The model under review builds one solid part; all positions refer to its coordinate system, in mm. A direction names the side the tool comes from. Round coordinates to 2 decimals unless told otherwise and drop trailing zeros. Order: outer loops, then holes, each group sorted by start corner. A loop starts at its lowest first (then second) coordinate and runs counter-clockwise, first axis right, second up. Notation, with made-up numbers: M 1,51 L 6,51 A17 cw 6,77 Z; hole C 65.5,63.25 d11. An arc over 180 degrees is marked long. Answer as a JSON object with one key per item and string values. Group by question number.
1. Add section A-A on z = -39.2. State the section outline as (x, y) points.
2. Clearance check with flat-ended pins moving along their axes: P1, Ø6, axis at y = 17.5, z = -7.5, coming from the +X side; P2, Ø1.5, axis at x = 28, z = 1.5, coming from the +Y side; P3, Ø7, axis at x = 1, z = -16, coming from the -Y side; P4, Ø4, axis at y = 1.96, z = -39.2, coming from the -X side. State where each tip first meets the part, or that it passes through.
3. To check wall thickness, follow probe 1 along Y at (x, z) = (-11, -8); probe 2 along Y at (x, z) = (-11, -39); probe 3 along X at (y, z) = (3.5, -15.5). State the ranges of each line that lie inside material, in increasing order. Write a range as [from, to].
4. Mouldability with a two-part tool opening along Y and no side actions: class faces 1 (the face through (1, 25, 3)), 2 (the face through (24, 40.963, 1)), 3 (the face through (-0.37, 32.34, 1.99)), 4 (the face through (7.39, -1.15, 1.48)) as released by +Y, released by -Y, zero draft, split by the parting line, or undercut.
5. Add section B-B on y = 34. State the section outline as (x, z) points, and give its area (3 significant figures).
6. Add section D-D on z = -20. State the section outline as (x, y) points, and give its area (3 significant figures).
7. Machinability: for faces 5 (the face through (-3, 40.963, -7)), 6 (the face through (4.04, 23.95, 1.48)), which of the approach directions +Z, -Z, +X, -X, +Y, -Y give a long, thin tool a straight path to every point of the face, cutting with its end or side? Answer none if there is none.
8. Add section C-C on x = 0. State the section outline as (y, z) points.
```python
from build123d import *

# Parameters (mm, degrees)
SKETCH_1_R          = 1.7
EXTRUDE_1_DEPTH     = 3
SKETCH_2_W          = 3.161086378
SKETCH_2_H          = 42
EXTRUDE_2_DEPTH     = 45
SKETCH_3_R          = 1.7
SKETCH_3_R_2        = 13
CUT_EXTRUDE_1_DEPTH = 45
SKETCH_4_R          = 14.357158039
CUT_EXTRUDE_2_DEPTH = 5
SKETCH_5_W          = 3.756135355
SKETCH_5_H          = 42.889588607
CUT_EXTRUDE_3_DEPTH = 5
CHAMFER_1_SIZE      = 1
EXTRUDE_3_DEPTH     = 3
EXTRUDE_4_DEPTH     = 3


with BuildPart() as part:
    # Эскиз1 → Бобышка-Вытянуть1 (new body)
    with BuildSketch(Plane.XY):
        Polygon((34, 31), (34, 34), (34, 37.963249048), (-1.7, 37.963249048), (-6, 37.963249048), (-12.575968026, 37.963249048), (-12.575968026, -4.036750952), (-6, -4.036750952), (5, -4.036750952), align=None)
        Circle(SKETCH_1_R, mode=Mode.SUBTRACT)
        with Locations((0, 34)):
            Circle(SKETCH_1_R, mode=Mode.SUBTRACT)
        with Locations((30, 34)):
            Circle(SKETCH_1_R, mode=Mode.SUBTRACT)
    extrude(amount=EXTRUDE_1_DEPTH)

    # Эскиз2 → Бобышка-Вытянуть2 (add)
    with BuildSketch(Plane(origin=(0, 0, 0), x_dir=(-1, 0, 0), z_dir=(0, 0, -1))):
        with Locations((10.995424837, 16.963249048)):
            Rectangle(SKETCH_2_W, SKETCH_2_H)
    extrude(amount=EXTRUDE_2_DEPTH)

    # Эскиз3 → Вырез-Вытянуть1 (cut)
    with BuildSketch(Plane(origin=(-9.414881648, 0, 0), x_dir=(0, 0, -1), z_dir=(1, 0, 0))):
        with Locations((8.2, 32.963249048)):
            Circle(SKETCH_3_R)
        with Locations((8.2, 1.963249048)):
            Circle(SKETCH_3_R)
        with Locations((39.2, 1.963249048)):
            Circle(SKETCH_3_R)
        with Locations((39.2, 32.963249048)):
            Circle(SKETCH_3_R)
        with Locations((23.7, 17.463249048)):
            Circle(SKETCH_3_R_2)
    extrude(amount=-CUT_EXTRUDE_1_DEPTH, mode=Mode.SUBTRACT)

    # Эскиз4 → Вырез-Вытянуть2 (cut)
    with BuildSketch(Plane(origin=(0, 0, 0), x_dir=(-1, 0, 0), z_dir=(0, 0, -1))):
        with Locations((-15.336156096, 15.085397016)):
            Circle(SKETCH_4_R)
    extrude(amount=-CUT_EXTRUDE_2_DEPTH, mode=Mode.SUBTRACT)

    # Эскиз5 → Вырез-Вытянуть3 (cut)
    with BuildSketch(Plane(origin=(-9.414881648, 0, 0), x_dir=(0, 0, -1), z_dir=(1, 0, 0))):
        with Locations((45.97241361, 16.518454745)):
            Rectangle(SKETCH_5_W, SKETCH_5_H)
    extrude(amount=-CUT_EXTRUDE_3_DEPTH, mode=Mode.SUBTRACT)

    # Фаска1
    chamfer_1_edges = [part.edges().sort_by_distance(p)[0] for p in [
        (28.3, 34, 0),
        (-1.7, 34, 0),
        (-1.7, 0, 0),
    ]]
    chamfer(chamfer_1_edges, length=CHAMFER_1_SIZE)

    # Эскиз6 → Бобышка-Вытянуть3 (add)
    with BuildSketch(Plane(origin=(0, 37.963249048, 0), x_dir=(1, 0, 0), z_dir=(0, 1, 0))):
        Polygon((34, -3), (34, 0), (-9.414881648, 0), (-9.414881648, 44.094345932), (-12.575968026, 44.094345932), (-12.575968026, -3), align=None)
    extrude(amount=EXTRUDE_3_DEPTH)

    # Эскиз7 → Бобышка-Вытянуть4 (add)
    with BuildSketch(Plane(origin=(0, 40.963249048, 0), x_dir=(1, 0, 0), z_dir=(0, 1, 0))):
        Polygon((17.424031974, -3), (-12.575968026, -3), (-12.575968026, 27), align=None)
    extrude(amount=EXTRUDE_4_DEPTH)


solid = part.part
```
Recorded:
{
 "1": {"outline": "M -12.58,-4.04 L -9.41,-4.04 L -9.41,0.26 L -12.58,0.26 Z; M -12.58,3.66 L -9.41,3.66 L -9.41,31.26 L -12.58,31.26 Z; M -12.58,34.66 L -9.41,34.66 L -9.41,40.96 L -12.58,40.96 Z"},
 "2": {"P1": "stops at x = -9.41", "P2": "stops at y = 40.96", "P3": "stops at y = 40.96", "P4": "stops at x = -12.58"},
 "3": {"probe 1": "y = [-4.04, 0.28], [3.65, 31.28], [34.65, 43.96]", "probe 2": "y = [-4.04, 0.28], [3.65, 31.28], [34.65, 40.96]", "probe 3": "x = [-12.58, -9.41]"},
 "4": {"face 1": "zero draft", "face 2": "released by +Y", "face 3": "undercut", "face 4": "released by -Y"},
 "5": {"outline": "M -12.58,-44.09 L -9.41,-44.09 L -9.41,-40.55 L -12.58,-40.55 Z; M -12.58,-37.85 L -9.41,-37.85 L -9.41,-9.55 L -12.58,-9.55 Z; M -12.58,-6.85 L -9.41,-6.85 L -9.41,0 L -2.7,0 L -1.7,1 L -1.7,3 L -12.58,3 Z; M 1.7,1 L 2.7,0 L 27.3,0 L 28.3,1 L 28.3,3 L 1.7,3 Z; M 31.7,1 L 32.7,0 L 34,0 L 34,3 L 31.7,3 Z", "area": "240 mm²"},
 "6": {"outline": "M -12.58,-4.04 L -9.41,-4.04 L -9.41,5 L -12.58,5 Z; M -12.58,29.93 L -9.41,29.93 L -9.41,40.96 L -5.58,40.96 L -5.58,43.96 L -12.58,43.96 Z", "area": "84.5 mm²"},
 "7": {"face 5": "-Z, +X, -Y", "face 6": "+Z, -Z"},
 "8": {"outline": "M -4.04,0 L -2.7,0 L -1.7,1 L -1.7,3 L -4.04,3 Z; M 1.7,1 L 2.7,0 L 31.3,0 L 32.3,1 L 32.3,3 L 1.7,3 Z; M 35.7,1 L 36.7,0 L 40.96,0 L 40.96,-14.42 L 43.96,-14.42 L 43.96,3 L 35.7,3 Z"}
}
